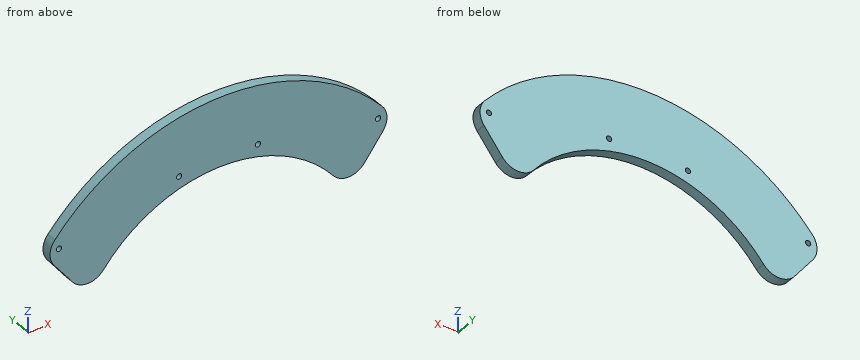
from build123d import *

# Parameters (mm, degrees)
SKETCH1_R           = 1.70053
BOSS_EXTRUDE1_DEPTH = 6.35


with BuildPart() as part:
    # Sketch1 → Boss-Extrude1 (new body)
    with BuildSketch(Plane(origin=(0, 0, 0), x_dir=(1, 0, 0), z_dir=(0, 1, 0))):
        with BuildLine():
            Line((-105.977429974, 26.723858277), (-94.097535909, 42.20603765))
            ThreePointArc((-94.097535909, 42.20603765), (-84.176111379, 47.17383179), (-74.137013371, 42.448352501))
            ThreePointArc((-74.137013371, 42.448352501), (0, 7.00024), (74.137013371, 42.448352501))
            ThreePointArc((74.137013371, 42.448352501), (84.176111379, 47.17383179), (94.097535909, 42.20603765))
            Line((94.097535909, 42.20603765), (105.977429974, 26.723858277))
            ThreePointArc((105.977429974, 26.723858277), (108.596043585, 18.608843232), (105.492026807, 10.666822942))
            ThreePointArc((105.492026807, 10.666822942), (0, -37.44976), (-105.492026807, 10.666822942))
            ThreePointArc((-105.492026807, 10.666822942), (-108.596043585, 18.608843232), (-105.977429974, 26.723858277))
        make_face()
        with Locations(Location((102.87, 17.39751111, 0), (0, 0, 270))):
            Circle(SKETCH1_R, mode=Mode.SUBTRACT)
        with Locations(Location((25.4, 2.54, 0), (0, 0, 270))):
            Circle(SKETCH1_R, mode=Mode.SUBTRACT)
        with Locations(Location((-102.87, 17.39751111, 0), (0, 0, 90))):
            Circle(SKETCH1_R, mode=Mode.SUBTRACT)
        with Locations(Location((-25.4, 2.54, 0), (0, 0, 90))):
            Circle(SKETCH1_R, mode=Mode.SUBTRACT)
    extrude(amount=BOSS_EXTRUDE1_DEPTH)


solid = part.part
Geometry check sheet. Reference: the model listing, model coordinates, mm. Round coordinates to 2 decimals unless told otherwise and drop trailing zeros. Order: outer loops, then holes, each group sorted by start corner. A loop starts at its lowest first (then second) coordinate and runs counter-clockwise, first axis right, second up. Notation, with made-up numbers: M 46,43 L 61,43 A16 cw 61,50 Z; hole C 27,13.25 d9. An arc over 180 degrees is marked long. Answer in a Markdown table with one row per item.
(1) Scan lines: probe 1 along X at (y, z) = (3.75, -2.54); probe 2 along Z at (x, y) = (-25.4, 4.25); probe 3 along X at (y, z) = (4, -3). Record each from-to range of solid material in increasing order. Write a range as from..to.
Responses:
| item | result |
|---|---|
| probe 1 | x = -97.85..-27.1, -23.7..23.7, 27.1..97.85 |
| probe 2 | z = -10.45..-4.24, -0.84..35.12 |
| probe 3 | x = -98.31..-27.04, -23.76..23.76, 27.04..98.31 |
(2) Sectioned sample at C-C, the plane x = 39.5. Record the cut outline in (y, z), and give its area (3 significant figures).
Responses:
| item | result |
|---|---|
| outline | M 0,-15.58 L 6.35,-15.58 L 6.35,31.75 L 0,31.75 Z |
| area | 301 mm² |
(3) Go/stop test with flat-tipped pins: P1, Ø3, axis at x = 102.87, z = -17.4, coming from the +Y side; P2, Ø3, axis at x = 30.5, y = 4, coming from the +Z side; P3, Ø1, axis at y = 2, z = 15, coming from the +X side; P4, Ø1, axis at y = 2.5, z = 15, coming from the -X side. Record where each tip stops, or that it passes through.
Responses:
| item | result |
|---|---|
| P1 | passes through |
| P2 | stops at z = 34.41 |
| P3 | stops at x = 76.72 |
| P4 | stops at x = -76.72 |
(4) Sectioned sample at A-A, the plane y = 1.5. Record the cut outline in (x, z), and give its area (3 significant figures).
Responses:
| item | result |
|---|---|
| outline | M -105.98,-26.72 L -94.1,-42.21 A12.7 ccw -74.14,-42.45 A95.25 cw 74.14,-42.45 A12.7 ccw 94.1,-42.21 L 105.98,-26.72 A12.7 ccw 105.49,-10.67 A139.7 ccw -105.49,-10.67 A12.7 ccw Z; hole C -102.87,-17.4 d3.4; hole C -25.4,-2.54 d3.4; hole C 25.4,-2.54 d3.4; hole C 102.87,-17.4 d3.4 |
| area | 10,100 mm² |
(5) Sectioned sample at D-D, the plane z = -29. Record the cut outline in (x, y), and give its area (3 significant figures).
Responses:
| item | result |
|---|---|
| outline | M -104.23,0 L -60.88,0 L -60.88,6.35 L -104.23,6.35 Z; M 60.88,0 L 104.23,0 L 104.23,6.35 L 60.88,6.35 Z |
| area | 550 mm² |
(6) Sectioned sample at B-B, the plane z = -37.5. Record the cut outline in (x, y), and give its area (3 significant figures).
Responses:
| item | result |
|---|---|
| outline | M -97.71,0 L -69.86,0 L -69.86,6.35 L -97.71,6.35 Z; M 69.86,0 L 97.71,0 L 97.71,6.35 L 69.86,6.35 Z |
| area | 354 mm² |
